Geometry check sheet. Reference: the model listing, model coordinates, mm. A direction names the side the tool comes from. Round coordinates to 2 decimals unless told otherwise and drop trailing zeros. Loops run counter-clockwise (first coordinate to the right, second up) from the corner with the lowest first, then second, coordinate; pieces in that order, holes last. Notation, with made-up numbers: (43.25, -25) -> (91.25, -25) arc R27 cw to (91.25, 11) -> close; hole circle Ø1 at (33.25, 11.5). An arc over 180 degrees is marked (long way). Use one line per item in the form item = value.
from build123d import *

# Parameters (mm, degrees)
SKETCH1_R           = 2
BOSS_EXTRUDE1_DEPTH = 1


with BuildPart() as part:
    # Sketch1 → Boss-Extrude1 (new body)
    with BuildSketch(Plane(origin=(0, 0, 0), x_dir=(1, 0, 0), z_dir=(0, 1, 0))):
        with BuildLine():
            Line((-20, 6), (-20, 11))
            ThreePointArc((-20, 11), (-18.828427125, 13.828427125), (-16, 15))
            Line((-16, 15), (0, 15))
            Line((0, 15), (7, 8))
            Line((7, 8), (16, 8))
            Line((16, 8), (16, 15))
            ThreePointArc((16, 15), (18.828427125, 13.828427125), (20, 11))
            Line((20, 11), (20, 3))
            Line((20, 3), (-5, 3))
            Line((-5, 3), (-5, -3))
            Line((-5, -3), (20, -3))
            Line((20, -3), (20, -11))
            ThreePointArc((20, -11), (18.828427125, -13.828427125), (16, -15))
            Line((16, -15), (16, -8))
            Line((16, -8), (7, -8))
            Line((7, -8), (0, -15))
            Line((0, -15), (-16, -15))
            ThreePointArc((-16, -15), (-18.828427125, -13.828427125), (-20, -11))
            Line((-20, -11), (-20, -6))
            ThreePointArc((-20, -6), (-14, 0), (-20, 6))
        make_face()
        with Locations(Location((-16, -11, 0), (0, 0, 270))):
            Circle(SKETCH1_R, mode=Mode.SUBTRACT)
        with Locations(Location((-16, 11, 0), (0, 0, 270))):
            Circle(SKETCH1_R, mode=Mode.SUBTRACT)
    extrude(amount=BOSS_EXTRUDE1_DEPTH)


solid = part.part
1. Section check C-C (z = 12.5). Record the boundary of the cut face in (x, y), then the cut area to 3 significant figures.
Return value:
outline = (-19.71, 0) -> (-17.32, 0) -> (-17.32, 1) -> (-19.71, 1) -> close; (-14.68, 0) -> (2.5, 0) -> (2.5, 1) -> (-14.68, 1) -> close; (16, 0) -> (19.71, 0) -> (19.71, 1) -> (16, 1) -> close
area = 23.3 mm2
2. Section check A-A (x = -2). Record the boundary of the cut face in (y, z).
Return value:
outline = (0, -15) -> (1, -15) -> (1, -3) -> (0, -3) -> close; (0, 3) -> (1, 3) -> (1, 15) -> (0, 15) -> close
3. Mould release check, pull along X, two halves, no side actions. Record for faces 1 (the cylindrical face through (18.859, 0.493, 13.797)), 2 (the flat face through (3.5, 0.5, -11.5)), 3 (the flat face through (-20, 0.5, 8.5)), 4 (the cylindrical face through (-14.017, 0.493, -11.26)): released by +X, released by -X, zero draft, split by the parting line, or undercut.
Return value:
face_1 = released by +X
face_2 = undercut
face_3 = released by -X
face_4 = undercut
4. Section check D-D (x = -15). Record the boundary of the cut face in (y, z), then the cut area to 3 significant figures.
Return value:
outline = (0, -15) -> (1, -15) -> (1, -12.73) -> (0, -12.73) -> close; (0, -9.27) -> (1, -9.27) -> (1, -3.32) -> (0, -3.32) -> close; (0, 3.32) -> (1, 3.32) -> (1, 9.27) -> (0, 9.27) -> close; (0, 12.73) -> (1, 12.73) -> (1, 15) -> (0, 15) -> close
area = 16.4 mm2
5. Section check B-B (y = 0.3). Record the boundary of the cut face in (x, z), then the cut area to 3 significant figures.
Return value:
outline = (-20, -11) arc R4 ccw to (-16, -15) -> (0, -15) -> (7, -8) -> (16, -8) -> (16, -15) arc R4 ccw to (20, -11) -> (20, -3) -> (-5, -3) -> (-5, 3) -> (20, 3) -> (20, 11) arc R4 ccw to (16, 15) -> (16, 8) -> (7, 8) -> (0, 15) -> (-16, 15) arc R4 ccw to (-20, 11) -> (-20, 6) arc R6 cw to (-20, -6) -> close; hole circle Ø4 at (-16, -11); hole circle Ø4 at (-16, 11)
area = 780 mm2
6. Tool access check on faces 5 (the flat face through (3.5, 0.5, 11.5)), 6 (the cylindrical face through (-18.797, 0.493, 13.859)), 7 (the flat face through (-5, 0.5, 0)). Record the directions out of +Z, -Z, +X, -X, +Y, -Y that give a thin tool (end or side, any length) a straight path to the whole face; none if there is none.
Return value:
face_5 = +Z, +Y, -Y
face_6 = +Z, -X, +Y, -Y
face_7 = +X, +Y, -Y
7. Gauge pin test, flat end, axial feed: pin 1 (0.5 mm diameter, centred on x = 6, y = 0.5, fed in from -Z). Record the tip position at first contact, or that the pin passes through.
Return value:
pin_1 = -9.25
8. Material ranges on line 1 along Z through (x, y) = (-3.5, 0.45); line 2 along X through (y, z) = (0.6, 11); line 3 along Z through (x, y) = (14, 0.9), recorded low to high.
Return value:
line_1 = -15 to -3, 3 to 15
line_2 = -20 to -18, -14 to 4, 16 to 20
line_3 = -8 to -3, 3 to 8
